Geometry: final body of the model. Coordinates: model frame, mm. A direction names the side the tool comes from. Round coordinates to 2 decimals unless told otherwise and drop trailing zeros. Order: outer loops, then holes, each group sorted by start corner. A loop starts at its lowest first (then second) coordinate and runs counter-clockwise, first axis right, second up. Notation, with made-up numbers: (30, -30) -> (36, -30) arc R10 ccw to (36, -16) -> close; hole circle Ø1 at (-9.75, 0). An arc over 180 degrees is marked (long way). Put each result on its own line as item: value.
```python
from build123d import *

# Parameters (mm, degrees)
F0_W     = 70
F0_H     = 10
F1_DEPTH = 30
F0_H_2   = 40
F2_DEPTH = 25
F3_R     = 5
F4_DEPTH = 55.001


with BuildPart() as f1:
    # F0 (on Right) → F1 (new body, symmetric)
    with BuildSketch(Plane.YZ):
        with Locations((0, 25)):
            Rectangle(F0_W, F0_H)
        with BuildLine():
            Line((-35, 20), (-35, 30))
            ThreePointArc((-35, 30), (-65, 0), (-35, -30))
            Line((-35, -30), (-35, -20))
            ThreePointArc((-35, -20), (-55, 0), (-35, 20))
        make_face()
        with BuildLine():
            ThreePointArc((35, -30), (65, 0), (35, 30))
            Line((35, 30), (35, 20))
            ThreePointArc((35, 20), (55, 0), (35, -20))
            Line((35, -20), (35, -30))
        make_face()
        with Locations((0, -25)):
            Rectangle(F0_W, F0_H)
    extrude(amount=F1_DEPTH, both=True)

    # F0 (on Right) → F2 (join, symmetric)
    with BuildSketch(Plane.YZ):
        with BuildLine():
            Line((-35, -20), (-35, 20))
            ThreePointArc((-35, 20), (-55, 0), (-35, -20))
        make_face()
        Rectangle(F0_W, F0_H_2)
        with BuildLine():
            ThreePointArc((35, -20), (55, 0), (35, 20))
            Line((35, 20), (35, -20))
        make_face()
    extrude(amount=F2_DEPTH, both=True)

    # F3 (on face) → F4 (cut, through all)
    with BuildSketch(Plane.YZ.offset(25)):
        with Locations((-35, 0)):
            Circle(F3_R)
        with Locations((35, 0)):
            Circle(F3_R)
    extrude(amount=-F4_DEPTH, mode=Mode.SUBTRACT)


solid = f1.part
```
1. Set-up query: faces 4 (the face through (28, 0, 20)), 5 (the face through (-27, -55, 0)), 6 (the face through (0, 0, -30)). Return all of +Z, -Z, +X, -X, +Y, -Y with unobstructed straight access to the full face (end or side cutting, diameter ignored); none if empty.
Ans:
face 4: +X
face 5: -X
face 6: -Z, +X, -X, +Y, -Y
2. Cut plane C-C on x = -10.5. Return loops of the section in (y, z), and give its area (3 significant figures).
Ans:
outline: (-35, -30) -> (35, -30) arc R30 ccw to (35, 30) -> (-35, 30) arc R30 ccw to start; hole circle Ø10 at (-35, 0); hole circle Ø10 at (35, 0)
area: 6,870 mm²
3. Cut plane A-A on z = 0. Return loops of the section in (x, y), and give its area (3 significant figures).
Ans:
outline: (-30, -65) -> (30, -65) -> (30, -55) -> (25, -55) -> (25, -40) -> (-25, -40) -> (-25, -55) -> (-30, -55) -> close; (-30, 55) -> (-25, 55) -> (-25, 40) -> (25, 40) -> (25, 55) -> (30, 55) -> (30, 65) -> (-30, 65) -> close; (-25, -30) -> (25, -30) -> (25, 30) -> (-25, 30) -> close
area: 5,700 mm²
4. Cut plane B-B on y = 10.5. Return loops of the section in (x, z).
Ans:
outline: (-30, -30) -> (30, -30) -> (30, -20) -> (25, -20) -> (25, 20) -> (30, 20) -> (30, 30) -> (-30, 30) -> (-30, 20) -> (-25, 20) -> (-25, -20) -> (-30, -20) -> close
5. Material intervals for probe 1 along Y at (x, z) = (0.5, 0.5); probe 2 along Z at (x, y) = (-9, 35); probe 3 along Y at (x, z) = (20.5, -3.5), sorted ascending.
Ans:
probe 1: -65 to -39.97, -30.03 to 30.03, 39.97 to 65
probe 2: -30 to -5, 5 to 30
probe 3: -64.8 to -38.57, -31.43 to 31.43, 38.57 to 64.8
6. Contact query for flat-ended pins moving along their axis: P1, Ø4, axis at y = -21, z = -9.5, coming from the +X side; P2, Ø12, axis at x = 0.5, z = 20.5, coming from the +Y side; P3, Ø16, axis at y = 35, z = 0, coming from the -X side. Output: stop coordinate, or through.
Ans:
P1: x = 25
P2: y = 61.26
P3: x = -25
7. Cut plane D-D on y = 36.5. Return loops of the section in (x, z).
Ans:
outline: (-30, -29.96) -> (30, -29.96) -> (30, -19.94) -> (25, -19.94) -> (25, -4.77) -> (-25, -4.77) -> (-25, -19.94) -> (-30, -19.94) -> close; (-30, 19.94) -> (-25, 19.94) -> (-25, 4.77) -> (25, 4.77) -> (25, 19.94) -> (30, 19.94) -> (30, 29.96) -> (-30, 29.96) -> close
8. Draft query along Y for faces 1 (the face through (-30, -0.9, 20.4)), 2 (the face through (0.42, 64.993, -0.66)), 3 (the face through (28, 0, -20)). Return one class per face: +Y half, -Y half, draft (parallel to the pull), parting line (faces both ways), or undercut.
Ans:
face 1: draft
face 2: +Y half
face 3: undercut
